For this review, take the finished solid that the model builds, in its own axes (mm). Round coordinates to 2 decimals unless told otherwise and drop trailing zeros. Order: outer loops, then holes, each group sorted by start corner. A loop starts at its lowest first (then second) coordinate and runs counter-clockwise, first axis right, second up. Notation, with made-up numbers: (41.25, 30.25) - (47.25, 30.25) arc R17 ccw to (47.25, 39.25) - close; hole circle Ø8 at (4.5, 15). An arc over 180 degrees is marked (long way). Write each question's results on one line, items separated by ' | '. Start each with the question number.
(1) Take a section at A-A, the plane y = 249. Give the boundary of the cut face in (x, z).
(2) Insertion check: pin 1 Ø3 at (y, z) = (848, 12) entering from -X; pin 2 Ø12 at (y, z) = (429.5, 7.5) entering from -X; pin 3 Ø3 at (y, z) = (30, 13.5) entering from +X. Each pin has a flat end and moves straight along its axis. Give the tip position at first contact, or say it passes through.
(3) For L1, parallel to X at y = 363, z = 5.5; L2, parallel to Z at x = 0.5, y = 761.5; L3, parallel to X at y = 203.5, z = -1, list the stretches that pass through material, from the lowest coordinate up. Write a range as from..to.
Solid Edge part; units mm, degrees
sketch "Sketch1" plane through (10.8674, 0, 10.8674) normal (0, -1, 0) x (1, 0, 0)
  circle A0 centre (-10.8674, -10.8674) radius 15
extrude "Protrusion1" add sketch "Sketch1" against normal blind 440
chamfer "Chamfer" distance 1 angle 45 1 edges at (-15, 0, 0)
sketch "Sketch2" plane through (0, 220.5, 15) normal (0, 0, 1) x (0, -1, 0)
  line L0 (173.5, -4) -> (210.5, -4)
  arc A0 (210.5, 4) -> (210.5, -4) centre (210.5, 0) cw
  line L1 (210.5, 4) -> (173.5, 4)
  arc A1 (173.5, 4) -> (173.5, -4) centre (173.5, 0) ccw
extrude "KeySlot_Wheel_Hub" cut sketch "Sketch2" against normal blind 4
mirror "Mirror1" about plane through (0, 440, 0) normal (0, 1, 0) of "Protrusion1", "KeySlot_Wheel_Hub"
properties material "Steel"
Results below:
1) outline: circle Ø30 at (0, 0)
2) pin 1: stops at x = -10.71 | pin 2: stops at x = -14.92 | pin 3: stops at x = 9
3) L1: x = -13.96..13.96 | L2: z = -14.99..14.99 | L3: x = -14.97..14.97
